from build123d import *

# Parameters (mm, degrees)
SKETCH_2_W           = 30.5
SKETCH_2_H           = 20.5
SKETCH_2_W_2         = 22.5
SKETCH_2_H_2         = 12.5
EXTRUDE_1_DEPTH      = 12
SKETCH_3_W           = 2.75
SKETCH_3_H           = 10
EXTRUDE_2_DEPTH      = 3
SKETCH_4_W           = 4.940698383
SKETCH_4_H           = 10
CUT_EXTRUDE_1_DEPTH  = 9
EXTRUDE_3_DEPTH      = 20
EXTRUDE_4_REACH      = 38.805
SKETCH_7_R           = 1.252665059
CUT_EXTRUDE_2_DEPTH  = 41.374032496
SKETCH_8_W           = 10
SKETCH_8_H           = 10
CUT_EXTRUDE_3_DEPTH  = 18
SKETCH_10_W          = 23.106147985
SKETCH_10_H          = 7.754593222
CUT_EXTRUDE_4_DEPTH  = 42.146840705
SKETCH_11_R          = 1.5
CUT_EXTRUDE_5_DEPTH  = 44.934610502
CUT_EXTRUDE_6_REACH  = 60.181
SKETCH_12_W          = 11
SKETCH_12_H          = 11
SKETCH_13_W          = 23.5
SKETCH_13_H          = 13.5
CUT_EXTRUDE_7_DEPTH  = 42.146840705
SKETCH_14_W          = 9.129424231
SKETCH_14_H          = 10.218893611
CUT_EXTRUDE_8_DEPTH  = 42.146840705
SKETCH_15_W          = 55
SKETCH_15_H          = 30
EXTRUDE_5_DEPTH      = 12
CUT_EXTRUDE_9_DEPTH  = 43.579337712
SKETCH_18_R          = 2.5
CUT_EXTRUDE_10_DEPTH = 43.579337712
CUT_EXTRUDE_11_DEPTH = 43.579337712
CUT_EXTRUDE_12_REACH = 48.136
CUT_EXTRUDE_13_REACH = 44.579
SKETCH_21_R          = 1.5


with BuildPart() as part:
    # 草图2 → 凸台-拉伸1 (new body)
    with BuildSketch(Plane.XY):
        Rectangle(SKETCH_2_W, SKETCH_2_H)
        Rectangle(SKETCH_2_W_2, SKETCH_2_H_2, mode=Mode.SUBTRACT)
    extrude(amount=EXTRUDE_1_DEPTH)

    # 草图3 → 凸台-拉伸2 (add)
    with BuildSketch(Plane.XY.offset(12)):
        with Locations((-16.625, 0)):
            Rectangle(SKETCH_3_W, SKETCH_3_H)
    extrude_2 = extrude(amount=-EXTRUDE_2_DEPTH)

    # 镜向1: 凸台-拉伸2 across plane
    add(extrude_2.mirror(Plane(origin=(0, 0, 0), x_dir=(0, 0, 1), z_dir=(1, 0, 0))))

    # 草图4 → 切除-拉伸1 (cut)
    with BuildSketch(Plane(origin=(0, 0, 0), x_dir=(-1, 0, 0), z_dir=(0, 0, -1))):
        with Locations((15.220349192, 0)):
            Rectangle(SKETCH_4_W, SKETCH_4_H)
    cut_extrude_1 = extrude(amount=-CUT_EXTRUDE_1_DEPTH, mode=Mode.SUBTRACT)

    # 镜向2: 切除-拉伸1 across plane
    add(cut_extrude_1.mirror(Plane(origin=(0, 0, 0), x_dir=(0, 0, 1), z_dir=(1, 0, 0))), mode=Mode.SUBTRACT)

    # 草图5 → 凸台-拉伸3 (add)
    with BuildSketch(Plane.ZY.offset(18)):
        Polygon((12, 10.25), (12, 5), (12, -5), (12, -10.25), (0, -10.25), (0, -5), (0, 5), (0, 10.25), align=None)
    extrude(amount=EXTRUDE_3_DEPTH)

    # 草图6 → 凸台-拉伸4 (add, up to next)
    with BuildSketch(Plane.ZY.offset(15.25), mode=Mode.PRIVATE) as extrude_4_sk1:
        Polygon((12, -5), (9, -5), (0, -5), (0, -10.25), (12, -10.25), align=None)
    extrude_4_tool1 = extrude(extrude_4_sk1.sketch, amount=EXTRUDE_4_REACH, mode=Mode.PRIVATE) - part.part
    extrude_4 = extrude_4_tool1.solids().sort_by_distance((-15.25, -7.625, 6))[0]
    add(extrude_4)

    # 镜向3: 凸台-拉伸4 across plane
    add(extrude_4.mirror(Plane.ZX))

    # 草图7 → 切除-拉伸2 (cut, through all)
    with BuildSketch(Plane(origin=(0, 0, 9), x_dir=(-1, 0, 0), z_dir=(0, 0, -1))):
        with Locations((15.487865972, 2.296552608)):
            Circle(SKETCH_7_R)
    cut_extrude_2 = extrude(amount=-CUT_EXTRUDE_2_DEPTH, mode=Mode.SUBTRACT)

    # 草图8 → 切除-拉伸3 (cut)
    with BuildSketch(Plane.ZY.offset(38)):
        with Locations((6, 0)):
            Rectangle(SKETCH_8_W, SKETCH_8_H)
    extrude(amount=-CUT_EXTRUDE_3_DEPTH, mode=Mode.SUBTRACT)

    # 草图10 → 切除-拉伸4 (cut, through all)
    with BuildSketch(Plane(origin=(0, 0, 0), x_dir=(-1, 0, 0), z_dir=(0, 0, -1))):
        with Locations((31.553073992, 12.127296611)):
            Rectangle(SKETCH_10_W, SKETCH_10_H)
    cut_extrude_4 = extrude(amount=-CUT_EXTRUDE_4_DEPTH, mode=Mode.SUBTRACT)

    # 镜向4: 切除-拉伸4 across plane
    add(cut_extrude_4.mirror(Plane.ZX), mode=Mode.SUBTRACT)

    # 草图11 → 切除-拉伸5 (cut, through all)
    with BuildSketch(Plane.XZ.offset(8.25)):
        with Locations(Location((-28, 6, 0), (0, 0, 270))):
            Circle(SKETCH_11_R)
    extrude(amount=-CUT_EXTRUDE_5_DEPTH, mode=Mode.SUBTRACT)

    # 镜向5: 切除-拉伸2 across plane
    add(cut_extrude_2.mirror(Plane(origin=(0, 0, 0), x_dir=(0, 0, 1), z_dir=(1, 0, 0))), mode=Mode.SUBTRACT)

    # 切除-拉伸6: up to this face of the body (flat: up to its plane)
    cut_extrude_6_end = Plane(part.part.faces().sort_by_distance((-20, 0, 6))[0])
    # 草图12 → 切除-拉伸6 (cut, up to the picked face)
    with BuildSketch(Plane.ZY.offset(38), mode=Mode.PRIVATE) as cut_extrude_6_sk1:
        with Locations((6, 0)):
            Rectangle(SKETCH_12_W, SKETCH_12_H)
    cut_extrude_6_tool1 = split(extrude(cut_extrude_6_sk1.sketch, amount=-CUT_EXTRUDE_6_REACH, mode=Mode.PRIVATE), bisect_by=cut_extrude_6_end, keep=Keep.BOTH, mode=Mode.PRIVATE)
    add(cut_extrude_6_tool1.solids().sort_by(Axis((-38, 0, 6), (1, 0, 0)))[0], mode=Mode.SUBTRACT)

    # 草图13 → 切除-拉伸7 (cut, through all)
    with BuildSketch(Plane.XY.offset(12)):
        Rectangle(SKETCH_13_W, SKETCH_13_H)
    extrude(amount=-CUT_EXTRUDE_7_DEPTH, mode=Mode.SUBTRACT)

    # 草图14 → 切除-拉伸8 (cut, through all)
    with BuildSketch(Plane.XY.offset(12)):
        with Locations((13.435287884, 0.109446806)):
            Rectangle(SKETCH_14_W, SKETCH_14_H)
    extrude(amount=-CUT_EXTRUDE_8_DEPTH, mode=Mode.SUBTRACT)

    # 草图15 → 凸台-拉伸5 (add)
    with BuildSketch(Plane.XY.offset(12)):
        with Locations((7.5, 0)):
            Rectangle(SKETCH_15_W, SKETCH_15_H)
    extrude(amount=-EXTRUDE_5_DEPTH)

    # 草图17 → 切除-拉伸9 (cut, through all)
    with BuildSketch(Plane.XY.offset(12)):
        Polygon((35, -5), (35, 5), (31, 5), (31, 10.4), (-10, 10.4), (-10, -10.4), (31, -10.4), (31, -5), align=None)
    extrude(amount=-CUT_EXTRUDE_9_DEPTH, mode=Mode.SUBTRACT)

    # 草图18 → 切除-拉伸10 (cut, through all)
    with BuildSketch(Plane(origin=(0, 0, 0), x_dir=(-1, 0, 0), z_dir=(0, 0, -1))):
        with Locations((15, -5)):
            Circle(SKETCH_18_R)
    cut_extrude_10 = extrude(amount=-CUT_EXTRUDE_10_DEPTH, mode=Mode.SUBTRACT)

    # 镜向6: 切除-拉伸10 across plane
    add(cut_extrude_10.mirror(Plane.ZX), mode=Mode.SUBTRACT)

    # 草图19 → 切除-拉伸11 (cut, through all)
    with BuildSketch(Plane(origin=(0, 0, 0), x_dir=(-1, 0, 0), z_dir=(0, 0, -1))):
        Polygon((20, 8.25), (14.491422615, 15), (20, 15), align=None)
    cut_extrude_11 = extrude(amount=-CUT_EXTRUDE_11_DEPTH, mode=Mode.SUBTRACT)

    # 镜向7: 切除-拉伸11 across plane
    add(cut_extrude_11.mirror(Plane.ZX), mode=Mode.SUBTRACT)

    # 草图20 → 切除-拉伸12 (cut, up to next)
    with BuildSketch(Plane(origin=(0, 8.25, 0), x_dir=(1, 0, 0), z_dir=(0, 1, 0)), mode=Mode.PRIVATE) as cut_extrude_12_sk1:
        Polygon((-26.267949192, -3), (-29.732050808, -3), (-31.464101615, -6), (-29.732050808, -9), (-26.267949192, -9), (-24.535898385, -6), align=None)
    cut_extrude_12_tool1 = extrude(cut_extrude_12_sk1.sketch, amount=-CUT_EXTRUDE_12_REACH, mode=Mode.PRIVATE) & part.part
    add(cut_extrude_12_tool1.solids().sort_by_distance((-28, 8.25, 6))[0], mode=Mode.SUBTRACT)

    # 草图21 → 切除-拉伸13 (cut, up to next)
    with BuildSketch(Plane.XY.offset(12), mode=Mode.PRIVATE) as cut_extrude_13_sk1:
        with Locations((-24, 0)):
            Circle(SKETCH_21_R)
    cut_extrude_13_tool1 = extrude(cut_extrude_13_sk1.sketch, amount=-CUT_EXTRUDE_13_REACH, mode=Mode.PRIVATE) & part.part
    add(cut_extrude_13_tool1.solids().sort_by_distance((-24, 0, 12))[0], mode=Mode.SUBTRACT)


solid = part.part
Here's how the part is built. I have some questions about the finished solid (model axes, mm). A direction names the side the tool comes from. Round coordinates to 2 decimals unless told otherwise and drop trailing zeros. Write each loop counter-clockwise with the first axis right and the second up, starting at its lowest first coordinate (ties: lowest second). Pieces come first, ordered by that corner, then holes.
1. Suppose I cut it at C-C (z = 10.5). List the corners of the cut face in (x, y) for me.
2. For faces 1 (the flat face through (-25.4, 6.9, 7.5)), 2 (the flat face through (-29, 0, 11.5)), 3 (the cylindrical face through (-25.5, 0.07, 11.75)), 4 (the flat face through (33, -5, 6)), which set-ups out of +Z, -Z, +X, -X, +Y, -Y let a thin tool reach every point of the face, with its end or its side?
3. Suppose I cut it at B-B (y = 0). List the corners of the cut face in (x, z) for me, and give its area (4 significant figures).
4. Will these pins go through, and if not, where does the flat tip stop? pin 1 Ø5 at (x, z) = (-28, 6) entering from +Y; pin 2 Ø3.5 at (x, z) = (-32, 7.5) entering from -Y; pin 3 Ø5.5 at (x, z) = (-26, 4) entering from +Y.
5. Suppose I cut it at A-A (x = 19.5). List the corners of the cut face in (y, z) for me.
6. I need wall thicknesses on L1, parallel to Y at x = -24, z = 11.75; L2, parallel to Y at x = -9, z = 8.75; L3, parallel to Y at x = -15, z = 4.5. Which ranges of each line are inside material? Lowest first, please.
7. Suppose I cut it at D-D (x = -33). List the corners of the cut face in (y, z) for me.
8. If we mould it in two halves opening along Y, with no side actions, what happens to faces 5 (the flat face through (11, 10.4, 6)), 6 (the flat face through (-30.6, 6.9, 7.5)), 7 (the flat face through (-17.28, -11.58, 5.92)), 8 (the flat face through (-30.9, 8.25, 4.6))? For each: released by +Y, released by -Y, zero draft, split by the parting line, or undercut.
Answer sheet:
1. outline: (-38, -8.25) - (-20, -8.25) - (-14.49, -15) - (35, -15) - (35, -5) - (31, -5) - (31, -10.4) - (-10, -10.4) - (-10, 10.4) - (31, 10.4) - (31, 5) - (35, 5) - (35, 15) - (-14.49, 15) - (-20, 8.25) - (-38, 8.25) - (-38, 5.5) - (-20, 5.5) - (-20, -5.5) - (-38, -5.5) - close; hole circle Ø5 at (-15, -5); hole circle Ø5 at (-15, 5)
2. face 1: +Y
2. face 2: -X
2. face 3: +Z
2. face 4: +Z, -Z, +X
3. outline: (-38, 0) - (-10, 0) - (-10, 12) - (-22.5, 12) - (-22.5, 11.5) - (-20, 11.5) - (-20, 0.5) - (-38, 0.5) - close; (-38, 11.5) - (-25.5, 11.5) - (-25.5, 12) - (-38, 12) - close
3. area: 136.5 mm2
4. pin 1: stops at y = -5.5
4. pin 2: stops at y = -8.25
4. pin 3: stops at y = 8.25
5. outline: (-15, 0) - (-10.4, 0) - (-10.4, 12) - (-15, 12) - close; (10.4, 0) - (15, 0) - (15, 12) - (10.4, 12) - close
6. L1: y = -8.25 to -1.5, 1.5 to 8.25
6. L2: y = -15 to -10.4, 10.4 to 15
6. L3: y = -14.38 to -7.5, -2.5 to 2.5, 7.5 to 14.38
7. outline: (-8.25, 0) - (8.25, 0) - (8.25, 12) - (-8.25, 12) - close; hole (-5.5, 0.5) - (5.5, 0.5) - (5.5, 11.5) - (-5.5, 11.5) - close
8. face 5: undercut
8. face 6: zero draft
8. face 7: released by -Y
8. face 8: released by +Y
